```python
from build123d import *

# Parameters (mm, degrees)
CROQUIS1_W              = 224
CROQUIS1_H              = 180
SALIENTE_EXTRUIR1_DEPTH = 9.525
CORTAR_EXTRUIR1_DEPTH   = 12.7
REDONDEO1_R             = 5
CROQUIS3_R              = 8.73125
CORTAR_EXTRUIR2_DEPTH   = 13


with BuildPart() as part:
    # Croquis1 → Saliente-Extruir1 (new body)
    with BuildSketch(Plane.XY):
        with Locations((112, -90)):
            Rectangle(CROQUIS1_W, CROQUIS1_H)
    extrude(amount=SALIENTE_EXTRUIR1_DEPTH)

    # Croquis2 → Cortar-Extruir1 (cut)
    with BuildSketch(Plane.XY.offset(9.525)):
        Polygon((84, 0), (84, -118), (140, -118), (140, 0), (112, 0), align=None)
    extrude(amount=-CORTAR_EXTRUIR1_DEPTH, mode=Mode.SUBTRACT)

    # Redondeo1
    redondeo1_edges = [part.edges().sort_by_distance(p)[0] for p in [
        (84, 0, 4.7625),
        (140, 0, 4.7625),
        (140, -118, 4.7625),
        (84, -118, 4.7625),
        (0, 0, 4.7625),
        (224, 0, 4.7625),
    ]]
    fillet(redondeo1_edges, radius=REDONDEO1_R)

    # Croquis3 → Cortar-Extruir2 (cut)
    with BuildSketch(Plane.XY.offset(9.525)):
        with Locations((177, -25)):
            Circle(CROQUIS3_R)
        with Locations((47, -25)):
            Circle(CROQUIS3_R)
        with Locations((47, -155)):
            Circle(CROQUIS3_R)
        with Locations((177, -155)):
            Circle(CROQUIS3_R)
    extrude(amount=-CORTAR_EXTRUIR2_DEPTH, mode=Mode.SUBTRACT)


solid = part.part
```
Work out the finished part from the listing and answer in its coordinate system (mm). A direction names the side the tool comes from. Give positions to 0.01 mm unless a question says otherwise; leave off trailing zeros. Loops run counter-clockwise (first coordinate to the right, second up) from the corner with the lowest first, then second, coordinate; pieces in that order, holes last. Notation, with made-up numbers: (-36, -30) -> (-23, -30) arc R17 cw to (-23, -22) -> close; hole circle Ø1 at (35, 43.5). An arc over 180 degrees is marked (long way). Write item = value, one per line. Start each with the question number.
(1) The mould has two halves that part along X. Classify faces 1 (the flat face through (0, -94, 5)), 2 (the cylindrical face through (138, -117, 5)), 3 (the cylindrical face through (168.277, -24.616, 4.829)), 4 (the flat face through (110, -180, 5)): +X half, -X half, draft (parallel to the pull), parting line (faces both ways), or undercut.
(2) Find section B-B on x = 177. Give the vertices of the cut face in (y, z) (3 decimals), and give its area (3 significant figures).
(3) Find section C-C on y = -61. Give the vertices of the cut face in (x, z) (3 decimals), and give its area (3 significant figures).
(4) Find the intervals of material crossed by probe 1 along Y at (x, z) = (177, 7.5); probe 2 along X at (y, z) = (-97, 0.75); probe 3 along X at (y, z) = (-17, 3.5), in increasing order. Write a range as from..to.
(5) Given pin 1 Ø15.5 at (x, y) = (177, -155) entering from +Z; pin 2 Ø12 at (x, y) = (85.5, -35.5) entering from +Z (3 decimals); pin 3 Ø5 at (x, z) = (100.5, 6) entering from +Y, each flat-ended and moving along its own axis, determine where each tip first touches the part or whether it passes through.
(6) Which of the six approach directions +Z, -Z, +X, -X, +Y, -Y give full straight-line access (tool end or side, diameter ignored) to faces 5 (the cylindrical face through (141, -2, 5)), 6 (the cylindrical face through (168.277, -154.616, 4.829))?
(7) Find section D-D on z = 4.25. Give the vertices of the cut face in (x, y).
(8) Find section A-A on y = -155. Give the vertices of the cut face in (x, z) (3 decimals), and give its area (3 significant figures).
From the geometry:
q1.face_1 = -X half
q1.face_2 = undercut
q1.face_3 = undercut
q1.face_4 = draft
q2.outline = (-180, 0) -> (-163.731, 0) -> (-163.731, 9.525) -> (-180, 9.525) -> close; (-146.269, 0) -> (-33.731, 0) -> (-33.731, 9.525) -> (-146.269, 9.525) -> close; (-16.269, 0) -> (0, 0) -> (0, 9.525) -> (-16.269, 9.525) -> close
q2.area = 1,380 mm^2
q3.outline = (0, 0) -> (84, 0) -> (84, 9.525) -> (0, 9.525) -> close; (140, 0) -> (224, 0) -> (224, 9.525) -> (140, 9.525) -> close
q3.area = 1,600 mm^2
q4.probe_1 = -180..-163.73, -146.27..-33.73, -16.27..0
q4.probe_2 = 0..84, 140..224
q4.probe_3 = 0..43.5, 50.5..84, 140..173.5, 180.5..224
q5.pin_1 = through
q5.pin_2 = 9.525
q5.pin_3 = -118
q6.face_5 = +Z, -Z, +Y
q6.face_6 = +Z, -Z
q7.outline = (0, -180) -> (224, -180) -> (224, -5) arc R5 ccw to (219, 0) -> (145, 0) arc R5 ccw to (140, -5) -> (140, -113) arc R5 cw to (135, -118) -> (89, -118) arc R5 cw to (84, -113) -> (84, -5) arc R5 ccw to (79, 0) -> (5, 0) arc R5 ccw to (0, -5) -> close; hole circle Ø17.46 at (47, -155); hole circle Ø17.46 at (47, -25); hole circle Ø17.46 at (177, -155); hole circle Ø17.46 at (177, -25)
q8.outline = (0, 0) -> (38.269, 0) -> (38.269, 9.525) -> (0, 9.525) -> close; (55.731, 0) -> (168.269, 0) -> (168.269, 9.525) -> (55.731, 9.525) -> close; (185.731, 0) -> (224, 0) -> (224, 9.525) -> (185.731, 9.525) -> close
q8.area = 1,800 mm^2
